Here's how the part is built. I have some questions about the finished solid (model axes, mm). A direction names the side the tool comes from. Coordinates: 2 decimals unless noted, no trailing zeros. Write each loop counter-clockwise with the first axis right and the second up, starting at its lowest first coordinate (ties: lowest second). Pieces come first, ordered by that corner, then holes. Notation, with made-up numbers: M -32,-39 L -5,-39 A6 cw -5,-35 Z; hole C -9,68 d2. An arc over 180 degrees is marked long. Use one line per item in the form item = value. Start each with the question number.
1. Thinking about a two-plate mould opening in Y: for faces 6 (the face through (-2.774, 23.296, 0.586)), 7 (the face through (5, 0, 12)), 8 (the face through (10, 3, 0)), which applies, released by +Y, released by -Y, zero draft, split by the parting line, or undercut?
2. On a 3-axis mill with a long thin cutter (end or side, diameter ignored), from which of +Z, -Z, +X, -X, +Y, -Y can I reach the whole of each face in a straight line? I mean faces 1 (the face through (-3, 9, -11)), 2 (the face through (-0.5, 13, 5.5)), 3 (the face through (-2, 11.834, 0)), 4 (the face through (7.1, 1.4, 1)), 5 (the face through (-0.51, 23.79, 0.65)). Say none if no direction works.
3. I want a section at A-A, the plane z = 0. List the corners of the cut face in (x, y) for me, plus the area to 3 significant figures.
4. I want a section at D-D, the plane z = 5.5. List the corners of the cut face in (x, y) for me, plus the area to 3 significant figures.
5. I want a section at B-B, the plane x = 5.5. List the corners of the cut face in (y, z) for me.
6. I'm going to push flat-ended pins straight in: pin 1 Ø1 at (x, z) = (-2.5, -10.5) entering from -Y; pin 2 Ø1 at (y, z) = (10, -11.5) entering from -X; pin 3 Ø1.8 at (x, y) = (0, 6.5) entering from -Z; pin 4 Ø4 at (y, z) = (16, 11) entering from -X. Where does each tip first touch, or does it pass through?
7. I want a section at C-C, the plane y = 5.5. List the corners of the cut face in (x, z) for me, plus the area to 3 significant figures.
8. Please list where these lines run through material, in increasing order: line 1 along Z through (x, y) = (8.5, 2.75); line 2 along Y through (x, z) = (-0.5, 0); line 3 along Y through (x, z) = (-1.75, 0). Write a range as [from, to].
from build123d import *

# Parameters (mm, degrees)
SCHIZZO2_W                     = 10
SCHIZZO2_H                     = 8
ESTRUSIONE_ESTRUSIONE1_DEPTH   = 2
ESTRUSIONE_ESTRUSIONE1_2_DEPTH = 2
ESTRUSIONE_ESTRUSIONE2_DEPTH   = 2
ESTRUSIONE_ESTRUSIONE3_DEPTH   = 26
TAGLIO_ESTRUSIONE1_DEPTH       = 34.763886032
TAGLIO_ESTRUSIONE1_DEPTH_BACK  = 34.763886032
TAGLIO_ESTRUSIONE2_DEPTH       = 32.990517073
TAGLIO_ESTRUSIONE2_DEPTH_BACK  = 32.990517073
SCHIZZO8_R                     = 2.5
ESTRUSIONE_ESTRUSIONE4_DEPTH   = 1
SCHIZZO11_W                    = 8
SCHIZZO11_H                    = 1
ESTRUSIONE_ESTRUSIONE5_DEPTH   = 4
ESTRUSIONE_ESTRUSIONE6_START   = -4.5
SCHIZZO12_R                    = 4.5
SCHIZZO12_R_2                  = 2.5
ESTRUSIONE_ESTRUSIONE6_DEPTH   = 4.5
ESTRUSIONE_ESTRUSIONE7_START   = -1
SCHIZZO13_R                    = 5
SCHIZZO13_R_2                  = 4.5
ESTRUSIONE_ESTRUSIONE7_DEPTH   = 1
TAGLIO_ESTRUSIONE3_START       = 12
SCHIZZO14_W                    = 1
SCHIZZO14_H                    = 4
TAGLIO_ESTRUSIONE3_DEPTH       = 44.990517073
ESTRUSIONE_ESTRUSIONE8_DEPTH   = 1


with BuildPart() as part:
    # Schizzo2 → Estrusione-Estrusione1 (new body)
    with BuildSketch(Plane(origin=(0, 0, 0), x_dir=(1, 0, 0), z_dir=(0, 1, 0))):
        with Locations((5, 12)):
            Rectangle(SCHIZZO2_W, SCHIZZO2_H)
    extrude(amount=ESTRUSIONE_ESTRUSIONE1_DEPTH)



with BuildPart() as body_2:
    # Schizzo2 → Estrusione-Estrusione1 2 (new body)
    with BuildSketch(Plane(origin=(0, 0, 0), x_dir=(1, 0, 0), z_dir=(0, 1, 0))):
        with Locations((5, -12)):
            Rectangle(SCHIZZO2_W, SCHIZZO2_H)
    extrude(amount=ESTRUSIONE_ESTRUSIONE1_2_DEPTH)


with BuildPart() as part_1:
    add(part.part)

    add(body_2.part)  # Estrusione-Estrusione2 merges body 2
    # Schizzo3 → Estrusione-Estrusione2 (add)
    with BuildSketch(Plane(origin=(0, 2, 0), x_dir=(1, 0, 0), z_dir=(0, 1, 0))):
        Polygon((0, -9), (10, -9), (10, -4), (4, -4), (4, -2.5), (10, -2.5), (10, 2.5), (4, 2.5), (4, 4), (10, 4), (10, 9), (0, 9), align=None)
    extrude(amount=ESTRUSIONE_ESTRUSIONE2_DEPTH)

    # Schizzo5 → Estrusione-Estrusione3 (add)
    with BuildSketch(Plane(origin=(0, 2, 0), x_dir=(1, 0, 0), z_dir=(0, 1, 0))):
        Polygon((-4, 12), (2, 12), (2, -12), (-4, -12), (-4, -10), (0, -10), (0, 10), (-4, 10), align=None)
    extrude(amount=ESTRUSIONE_ESTRUSIONE3_DEPTH)

    # Schizzo6 → Taglio-Estrusione1 (cut, two sides: drawn at the far end of the back side and taken through both)
    with BuildSketch(Plane(origin=(0, 0, 0), x_dir=(0, 0, -1), z_dir=(1, 0, 0)).offset(-TAGLIO_ESTRUSIONE1_DEPTH_BACK)):
        with BuildLine():
            Line((-12, 10), (-12, 28))
            Line((-12, 28), (12, 28))
            Line((12, 28), (12, 10))
            Line((12, 10), (6, 15.291502622))
            ThreePointArc((6, 15.291502622), (6.640310502, 19.165456154), (5, 22.732933549))
            Line((5, 22.732933549), (5, 23.732933549))
            ThreePointArc((5, 23.732933549), (0, 25.833954064), (-5, 23.732933549))
            Line((-5, 23.732933549), (-5, 22.732933549))
            ThreePointArc((-5, 22.732933549), (-6.640310502, 19.165456154), (-6, 15.291502622))
            Line((-6, 15.291502622), (-12, 10))
        make_face()
    extrude(amount=TAGLIO_ESTRUSIONE1_DEPTH + TAGLIO_ESTRUSIONE1_DEPTH_BACK, mode=Mode.SUBTRACT)

    # Schizzo8 → Taglio-Estrusione2 (cut, two sides: drawn at the far end of the back side and taken through both)
    with BuildSketch(Plane(origin=(0, 0, 0), x_dir=(0, 0, -1), z_dir=(1, 0, 0)).offset(-TAGLIO_ESTRUSIONE2_DEPTH_BACK)):
        with Locations((0, 18.833954064)):
            Circle(SCHIZZO8_R)
    extrude(amount=TAGLIO_ESTRUSIONE2_DEPTH + TAGLIO_ESTRUSIONE2_DEPTH_BACK, mode=Mode.SUBTRACT)

    # Schizzo9 → Estrusione-Estrusione4 (add, symmetric)
    with BuildSketch(Plane.XY):
        Polygon((8, 2), (6.5, 2), (6.5, 0.5), align=None)
    extrude(amount=ESTRUSIONE_ESTRUSIONE4_DEPTH, both=True)

    # Schizzo11 → Estrusione-Estrusione5 (add)
    with BuildSketch(Plane(origin=(0, 0, 0), x_dir=(0, 0, -1), z_dir=(1, 0, 0))):
        with Locations((0, 12.333954064)):
            Rectangle(SCHIZZO11_W, SCHIZZO11_H)
    extrude(amount=-ESTRUSIONE_ESTRUSIONE5_DEPTH)

    # Schizzo12 → Estrusione-Estrusione6 (add)
    with BuildSketch(Plane(origin=(0, 0, 0), x_dir=(0, 0, -1), z_dir=(1, 0, 0)).offset(ESTRUSIONE_ESTRUSIONE6_START)):
        with Locations((0, 18.833954064)):
            Circle(SCHIZZO12_R)
        with Locations((0, 18.833954064)):
            Circle(SCHIZZO12_R_2, mode=Mode.SUBTRACT)
    extrude(amount=ESTRUSIONE_ESTRUSIONE6_DEPTH)

    # Schizzo13 → Estrusione-Estrusione7 (add)
    with BuildSketch(Plane(origin=(0, 0, 0), x_dir=(0, 0, -1), z_dir=(1, 0, 0)).offset(ESTRUSIONE_ESTRUSIONE7_START)):
        with Locations((0, 18.833954064)):
            Circle(SCHIZZO13_R)
        with Locations((0, 18.833954064)):
            Circle(SCHIZZO13_R_2, mode=Mode.SUBTRACT)
    extrude(amount=ESTRUSIONE_ESTRUSIONE7_DEPTH)

    # Schizzo14 → Taglio-Estrusione3 (cut, through all)
    with BuildSketch(Plane.XY.offset(TAGLIO_ESTRUSIONE3_START)):
        with Locations((-3.5, 9.763834207)):
            Rectangle(SCHIZZO14_W, SCHIZZO14_H)
    extrude(amount=-TAGLIO_ESTRUSIONE3_DEPTH, mode=Mode.SUBTRACT)

    # Schizzo17 → Estrusione-Estrusione8 (add)
    with BuildSketch(Plane(origin=(0, 0, 0), x_dir=(0, 0, -1), z_dir=(1, 0, 0))):
        with BuildLine():
            Line((6, 15.291502622), (6.75, 14.630064794))
            ThreePointArc((6.75, 14.630064794), (5.555843379, 13.054148343), (4, 11.833954064))
            Line((4, 11.833954064), (4, 12.833954064))
            ThreePointArc((4, 12.833954064), (5.136905867, 13.951311731), (6, 15.291502622))
        make_face()
        with BuildLine():
            Line((-6.75, 14.630064794), (-6, 15.291502622))
            ThreePointArc((-6, 15.291502622), (-5.136905867, 13.951311731), (-4, 12.833954064))
            Line((-4, 12.833954064), (-4, 11.833954064))
            ThreePointArc((-4, 11.833954064), (-5.555843379, 13.054148343), (-6.75, 14.630064794))
        make_face()
    extrude(amount=-ESTRUSIONE_ESTRUSIONE8_DEPTH)


solid = part_1.part
Answer list:
q1.face_6 = undercut
q1.face_7 = released by -Y
q1.face_8 = zero draft
q2.face_1 = +Z, -Z, -X, +Y
q2.face_2 = +Z, -X, -Y
q2.face_3 = +Z, -Z, -X, -Y
q2.face_4 = +X, -X, -Y
q2.face_5 = -X
q3.outline = M -4.5,14.33 L -1,14.33 L -1,13.83 L 0,13.83 L 0,12.83 L -4,12.83 L -4,11.83 L 0,11.83 L 0,2 L 6.5,2 L 6.5,0.5 L 8,2 L 10,2 L 10,4 L 2,4 L 2,16.33 L -4.5,16.33 Z; M -4.5,21.33 L 2,21.33 L 2,25.83 L 0,25.83 L 0,23.83 L -1,23.83 L -1,23.33 L -4.5,23.33 Z
q3.area = 77.8 mm²
q4.outline = M -1,13 L 0,13 L 0,2 L 10,2 L 10,4 L 2,4 L 2,22.1 L 0,22.1 L 0,14.44 L -1,14.44 Z
q4.area = 57.6 mm²
q5.outline = M 0,-16 L 2,-16 L 2,-9 L 4,-9 L 4,-4 L 2,-4 L 2,-8 L 0,-8 Z; M 0,8 L 2,8 L 2,4 L 4,4 L 4,9 L 2,9 L 2,16 L 0,16 Z; M 2,-2.5 L 4,-2.5 L 4,2.5 L 2,2.5 Z
q6.pin_1 = 2
q6.pin_2 = -3
q6.pin_3 = -12
q6.pin_4 = through
q7.outline = M -4,-12 L 2,-12 L 2,12 L -4,12 L -4,10 L 0,10 L 0,-10 L -4,-10 Z
q7.area = 64.0 mm²
q8.line_1 = [-9, -4], [-2.5, 2.5], [4, 9]
q8.line_2 = [11.83, 12.83], [13.83, 16.33], [21.33, 23.83]
q8.line_3 = [11.83, 12.83], [14.33, 16.33], [21.33, 23.33]
